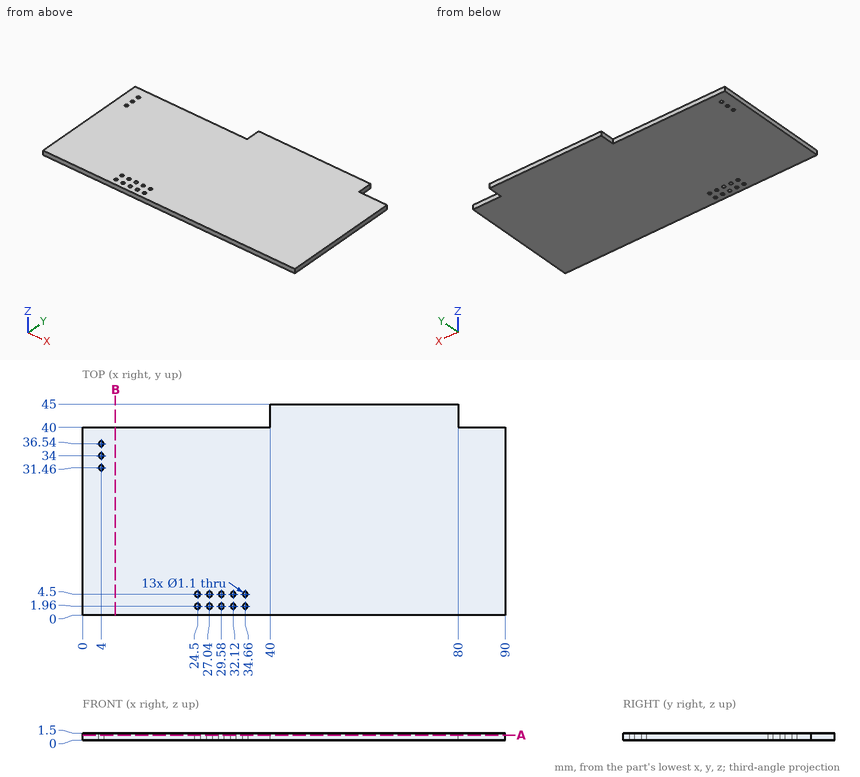
Here's the drawing with two shaded views (mm, measured from the low corner). I have some questions. Round coordinates to 2 decimals unless told otherwise and drop trailing zeros. Order: outer loops, then holes, each group sorted by start corner. A loop starts at its lowest first (then second) coordinate and runs counter-clockwise, first axis right, second up. Notation, with made-up numbers: M 83.25,12.5 L 110.25,12.5 A19 ccw 110.25,42.5 Z; hole C 35.5,0 d6. An arc over 180 degrees is marked long. Use CSV: the item, a comma, the result in double quotes.
1) I want a section at A-A (z = 1.1). Count the separate pieces of the cut face and the enclosed holes in it, then the cut area to 3 significant figures.
Taken from the geometry:
separate pieces,"1"
enclosed holes,"13"
area,"3,790 mm^2"
2) I'm going to push a flat-ended pin straight in: P1, Ø0.9, axis at x = 27.04, y = 4.5, coming from the -Z side. Where does the tip first touch, or does it pass through?
Taken from the geometry:
P1,"through"
3) I need wall thicknesses on line 1 along Y through (x, z) = (27.04, 1); line 2 along Y through (x, z) = (4, 0.95); line 3 along X through (y, z) = (34, 0.25). Which ranges of each line are inside material? Lowest first, please. Write a range as [from, to].
Taken from the geometry:
line 1,"[0, 1.41], [2.51, 3.95], [5.05, 40]"
line 2,"[0, 30.91], [32.01, 33.45], [34.55, 35.99], [37.09, 40]"
line 3,"[0, 3.45], [4.55, 90]"
4) I want a section at B-B (x = 7). List the corners of the cut face in (y, z) for me.
Taken from the geometry:
outline,"M 0,0 L 40,0 L 40,1.5 L 0,1.5 Z"
